Could you check a few things on this drawing? It's one solid part, dimensions in mm from its lowest x, y, z. A direction names the side the tool comes from. Coordinates: 2 decimals unless noted, no trailing zeros. Order: outer loops, then holes, each group sorted by start corner. A loop starts at its lowest first (then second) coordinate and runs counter-clockwise, first axis right, second up.
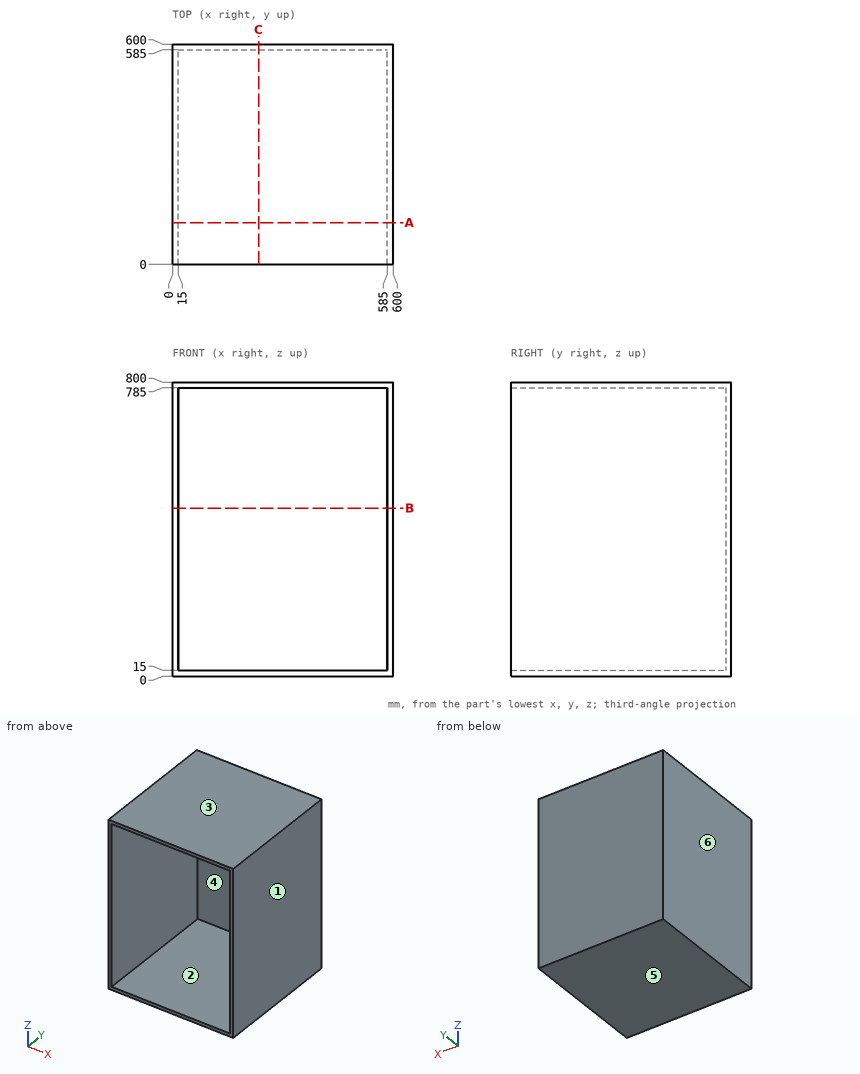
Q1. If we section it at A-A on y = 113.5: Write out the boundary of the cut face in (x, z), then the cut area to 3 significant figures.
Q2. For the marked faces 1 and 2, which set-ups out of +Z, -Z, +X, -X, +Y, -Y let a thin tool reach every point of the face, with its end or its side?
Q3. Will this pin go through, and if not, where does the flat tip stop? pin 1 (3 mm diameter, centred on x = 517.5, z = 548, fed in from -Y).
Q4. We'd pull the mould along Z, two halves only. Please class the marked faces 3, 4, 5 and 6: pulls with the +Z half, pulls with the -Z half, needs draft (parallel to the pull), parting line crosses it, or undercut.
Q5. I need wall thicknesses on L1, parallel to Z at x = 286.5, y = 297.5; L2, parallel to X at y = 151, z = 56; L3, parallel to Y at x = 292.5, z = 271.5. Which ranges of each line are inside material? Lowest first, please.
Q6. If we section it at C-C on x = 234: Write out the boundary of the cut face in (y, z).
Q7. If we section it at B-B on z = 457.5: Write out the boundary of the cut face in (x, y).
Reply:
1. outline: (0, 0) - (600, 0) - (600, 800) - (0, 800) - close; hole (15, 15) - (585, 15) - (585, 785) - (15, 785) - close
1. area: 41,100 mm2
2. face 1: +Z, -Z, +X, +Y, -Y
2. face 2: -Y
3. pin 1: stops at y = 585
4. face 3: pulls with the +Z half
4. face 4: undercut
4. face 5: pulls with the -Z half
4. face 6: needs draft
5. L1: z = 0 to 15, 785 to 800
5. L2: x = 0 to 15, 585 to 600
5. L3: y = 585 to 600
6. outline: (0, 0) - (600, 0) - (600, 800) - (0, 800) - (0, 785) - (585, 785) - (585, 15) - (0, 15) - close
7. outline: (0, 0) - (15, 0) - (15, 585) - (585, 585) - (585, 0) - (600, 0) - (600, 600) - (0, 600) - close
